Could you check a few things on this model? Use its own coordinates, in mm. A direction names the side the tool comes from. Coordinates: 2 decimals unless noted, no trailing zeros. Write each loop counter-clockwise with the first axis right and the second up, starting at its lowest first coordinate (ties: lowest second). Pieces come first, ordered by that corner, then holes.
```python
from build123d import *

# Parameters (mm, degrees)
F0_W     = 32.1596805006
F0_H     = 12.7692851238
F1_DEPTH = 25
F2_T     = -2.5


with BuildPart() as f1:
    # F0 (on Right) → F1 (new body)
    with BuildSketch(Plane.YZ):
        with Locations((-2.3078126833, 13.5815928224)):
            Rectangle(F0_W, F0_H)
        Polygon((-18.3876529336, 19.9662353843), (-33.5216186941, 19.9662353843), (-33.5216186941, -28.2732862979), (-18.3876529336, -28.2732862979), (-18.3876529336, 7.1969502605), align=None)
    extrude(amount=F1_DEPTH)

    # F2
    f2_openings = [f1.faces().sort_by_distance(p)[0] for p in [
        (12.5, 13.772028, 13.581593),
    ]]
    offset(amount=F2_T, openings=f2_openings, kind=Kind.INTERSECTION)


solid = f1.part
```
1. If we mould it in two halves opening along X, with no side actions, what happens to faces 4 (the face through (12, 13.772, 18)), 5 (the face through (0, -21, 2)), 6 (the face through (12, -31.022, -4)), 7 (the face through (25, -21, 2))? For each: pulls with the +X half, pulls with the -X half, needs draft (parallel to the pull), parting line crosses it, or undercut.
Verdict:
face 4: needs draft
face 5: pulls with the -X half
face 6: undercut
face 7: pulls with the +X half
2. I want a section at B-B on y = -5. Please give me the cut outline in (x, z).
Verdict:
outline: (0, 7.2) - (25, 7.2) - (25, 19.97) - (0, 19.97) - close; hole (2.5, 9.7) - (22.5, 9.7) - (22.5, 17.47) - (2.5, 17.47) - close
3. I want a section at A-A on z = -23. Please give me the cut outline in (x, y), plus the area to 3 significant figures.
Verdict:
outline: (0, -33.52) - (25, -33.52) - (25, -18.39) - (0, -18.39) - close; hole (2.5, -31.02) - (22.5, -31.02) - (22.5, -20.89) - (2.5, -20.89) - close
area: 176 mm2
4. On a 3-axis mill with a long thin cutter (end or side, diameter ignored), from which of +Z, -Z, +X, -X, +Y, -Y can I reach the whole of each face in a straight line? I mean faces 1 (the face through (12, -8, 17.466)), 2 (the face through (12, -18.388, -11)), 3 (the face through (12, -26, -25.773)). Say none if no direction works.
Verdict:
face 1: +Y
face 2: -Z, +X, -X, +Y
face 3: none
5. For pin 1 (1.5 mm diameter, centred on y = 7, z = 10, fed in from -X); pin 2 (12.5 mm diameter, centred on x = 15.5, y = -3, fed in from -Z); pin 3 (8 mm diameter, centred on x = 21, z = -12, fed in from +Y), each with a flat end and sliding along its axis, tell me the tip position at first contact or that it passes through.
Verdict:
pin 1: stops at x = 0
pin 2: stops at z = 7.2
pin 3: stops at y = -18.39
6. I want a section at D-D on z = 15. Please give me the cut outline in (x, y), plus the area to 3 significant figures.
Verdict:
outline: (0, -33.52) - (25, -33.52) - (25, 13.77) - (22.5, 13.77) - (22.5, -31.02) - (2.5, -31.02) - (2.5, 13.77) - (0, 13.77) - close
area: 286 mm2
7. Please list where these lines run through material, in increasing order: line 1 along Y through (x, z) = (8.5, -8.5); line 2 along Z through (x, y) = (21, -9.5); line 3 along X through (y, z) = (-25, -15).
Verdict:
line 1: y = -33.52 to -31.02, -20.89 to -18.39
line 2: z = 7.2 to 9.7, 17.47 to 19.97
line 3: x = 0 to 2.5, 22.5 to 25
8. I want a section at C-C on x = 12.5. Please give me the cut outline in (y, z), plus the area to 3 significant figures.
Verdict:
outline: (-33.52, -28.27) - (-18.39, -28.27) - (-18.39, 7.2) - (13.77, 7.2) - (13.77, 9.7) - (-20.89, 9.7) - (-20.89, -25.77) - (-31.02, -25.77) - (-31.02, 17.47) - (13.77, 17.47) - (13.77, 19.97) - (-33.52, 19.97) - close
area: 433 mm2
